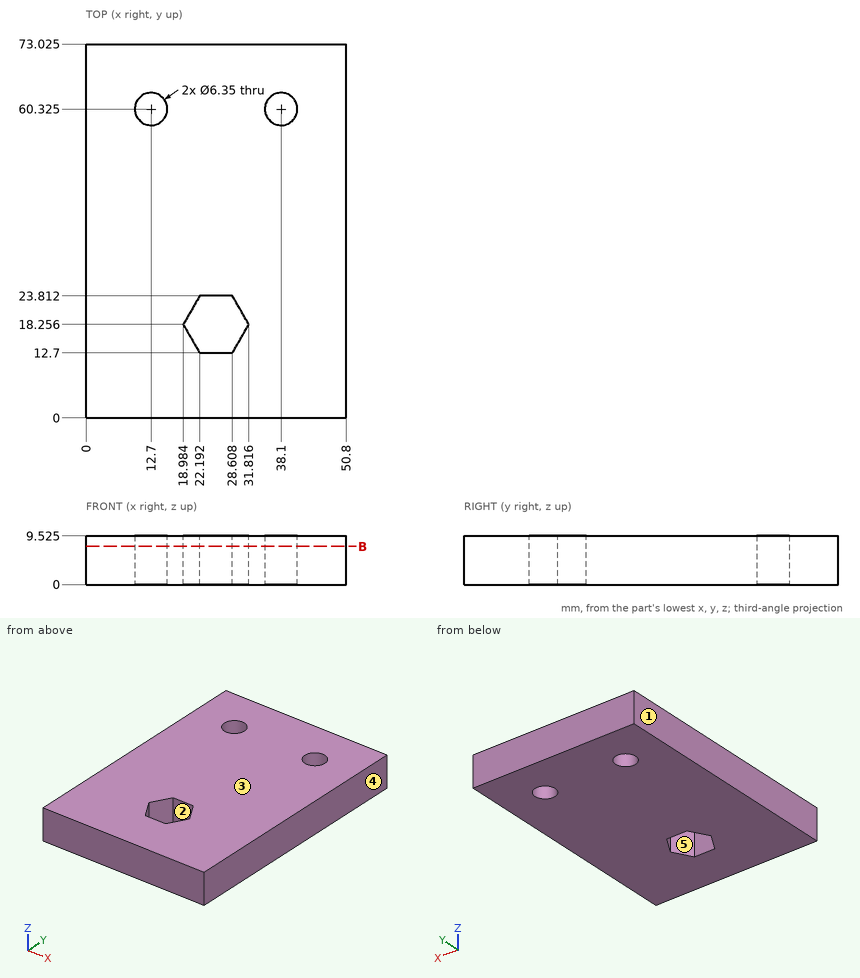
Can you work these out from the drawing? Everything is in mm from the part's minimum corner. A direction names the side the tool comes from. Round coordinates to 2 decimals unless told otherwise and drop trailing zeros.
1. Which directions (+Z, -Z, +X, -X, +Y, -Y) give clear straight access to the entire face, cutting with the end or side of a thin tool? Please do the marked faces 1 and 2.
Answer list:
face 1: +Z, -Z, -X, +Y, -Y
face 2: +Z, -Z
2. If I drill on line 1 along Y through (x, z) = (14.5, 4) (1 decimal); line 2 along Y through (x, z) = (41, 5.25) (1 decimal); line 3 along X through (y, z) = (23.5, 8), over which ranges is the centre line in solid material (lowest first)?
Answer list:
line 1: y = 0 to 57.7, 62.9 to 73
line 2: y = 0 to 59, 61.6 to 73
line 3: x = 0 to 22.01, 28.79 to 50.8
3. For P1, Ø10, axis at x = 12.7, y = 60.325, coming from the -Z side, with a flat end and sliding along its axis, tell me the tip position at first contact or that it passes through.
Answer list:
P1: stops at z = 0
4. If we section it at B-B on z = 7.5: Count the separate pieces of the cut face and the enclosed holes in it, plus the area to 3 significant figures.
Answer list:
separate pieces: 1
enclosed holes: 3
area: 3,540 mm2
5. We'd pull the mould along X, two halves only. Please class the marked faces 3, 4 and 5: +X half, -X half, draft (parallel to the pull), parting line (faces both ways), or undercut.
Answer list:
face 3: draft
face 4: +X half
face 5: undercut
